Can you work these out from the drawing? Everything is in mm from the part's minimum corner. Give positions to 0.01 mm unless a question says otherwise; leave off trailing zeros. Order: outer loops, then holes, each group sorted by start corner. A loop starts at its lowest first (then second) coordinate and runs counter-clockwise, first axis right, second up. Notation, with made-up numbers: M 15,-18.75 L 30,-18.75 A12 cw 30,-4.75 Z; hole C -5.5,26 d2. An arc over 180 degrees is marked long. Use a Markdown table: item, result. Add a question column.
Item 1: If we mould it in two halves opening along Y, with no side actions, what happens to the marked faces 1, 2, 3 and 4? For each: released by +Y, released by -Y, zero draft, split by the parting line, or undercut.
Item 2: Suppose I cut it at C-C on z = 11. Write out the boundary of the cut face in (x, y) (1 decimal).
Item 3: Suppose I cut it at A-A on x = 12. Write out the boundary of the cut face in (y, z).
Item 4: Suppose I cut it at B-B on y = 24.5. Write out the boundary of the cut face in (x, z) (1 decimal).
Item 5: If I drill on L1, parallel to Y at x = 20.5, z = 5; L2, parallel to Y at x = 32.5, z = 25; L3, parallel to X at y = 19.5, z = 43, over which ranges is the centre line in solid material (lowest first)? Write a range as from..to.
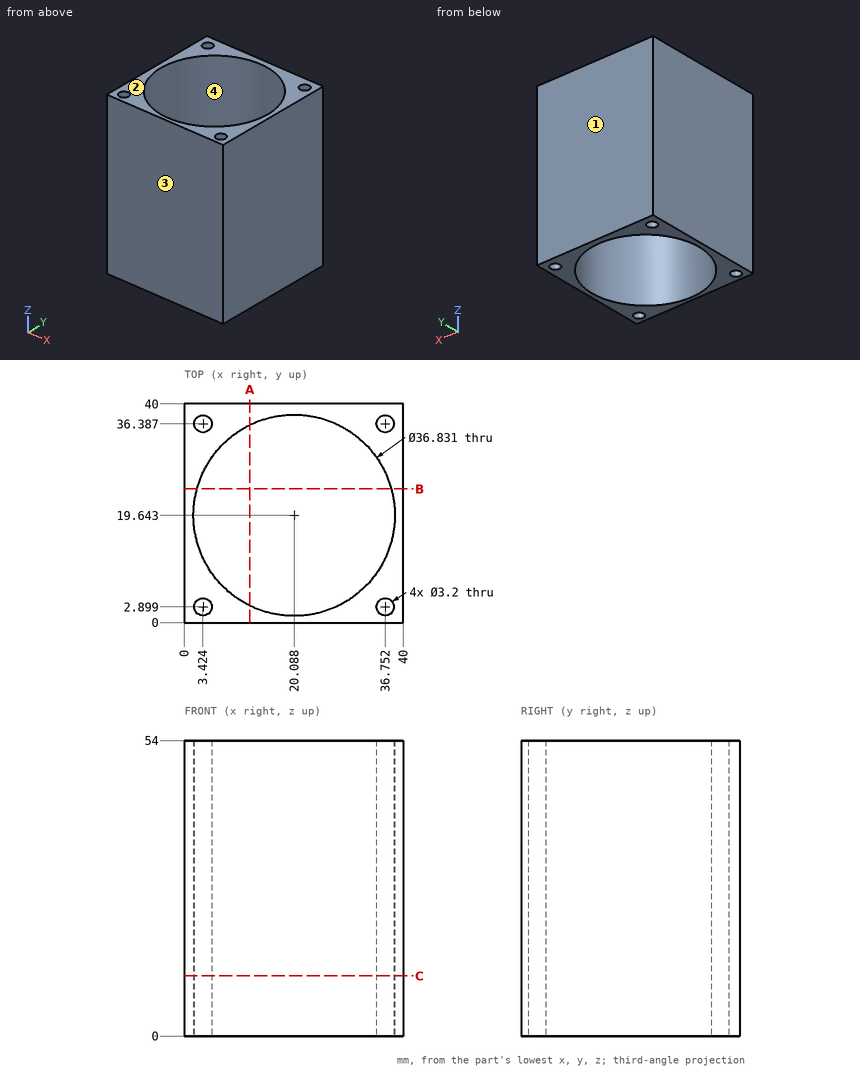
Findings below:
| question | item | result |
|---|---|---|
| 1 | face 1 | released by +Y |
| 1 | face 2 | zero draft |
| 1 | face 3 | released by -Y |
| 1 | face 4 | undercut |
| 2 | outline | M 0,0 L 40,0 L 40,40 L 0,40 Z; hole C 20.1,19.6 d36.8; hole C 3.4,2.9 d3.2; hole C 3.4,36.4 d3.2; hole C 36.8,2.9 d3.2; hole C 36.8,36.4 d3.2 |
| 3 | outline | M 0,0 L 3.1,0 L 3.1,54 L 0,54 Z; M 36.19,0 L 40,0 L 40,54 L 36.19,54 Z |
| 4 | outline | M 0,0 L 2.3,0 L 2.3,54 L 0,54 Z; M 37.9,0 L 40,0 L 40,54 L 37.9,54 Z |
| 5 | L1 | y = 0..1.23, 38.05..40 |
| 5 | L2 | y = 0..6.04, 33.25..40 |
| 5 | L3 | x = 0..1.67, 38.5..40 |
